Input: dimensioned drawing with shaded views. Units: mm. Origin: part minimum x, y, z. A direction names the side the tool comes from. Coordinates: 2 decimals unless noted, no trailing zeros. Write each loop counter-clockwise with the first axis right and the second up, starting at its lowest first coordinate (ties: lowest second). Pieces come first, ordered by that corner, then holes. Notation, with made-up numbers: M 15,84.5 L 38,84.5 A16 ccw 38,101.5 Z; hole C -16,75 d11. An arc over 180 degrees is marked long. Use one line per item in the form item = value.
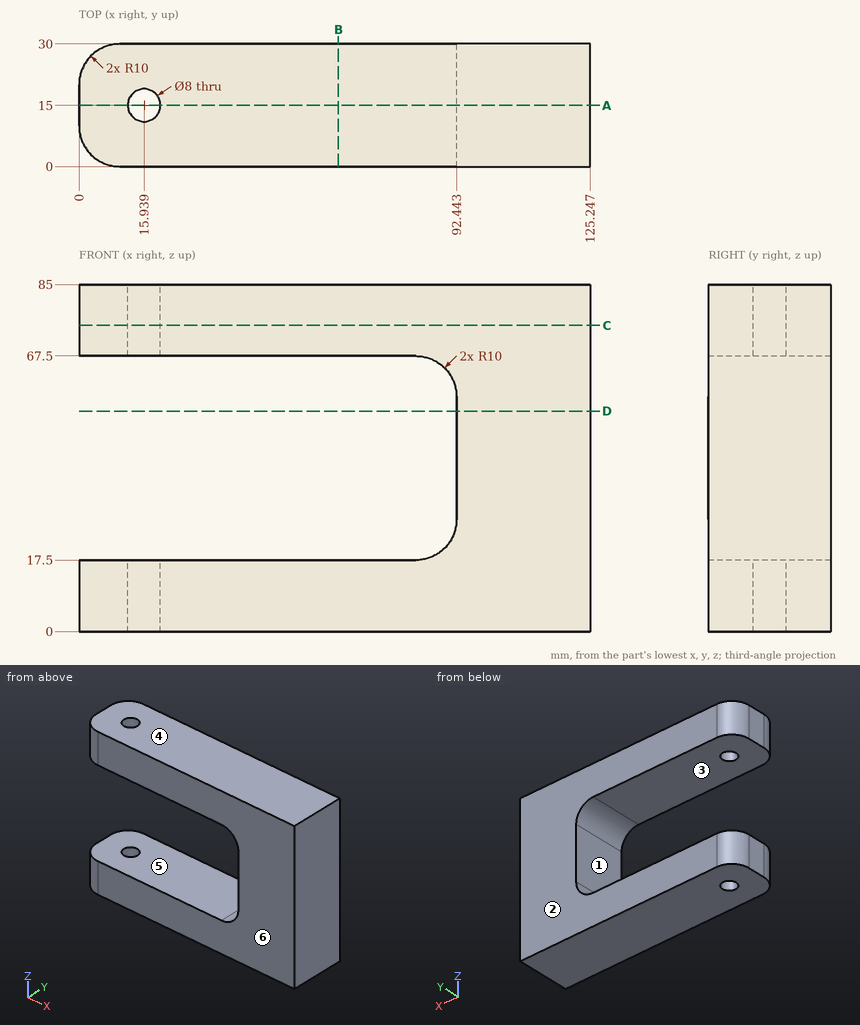
(1) Section query B-B on x = 63.5. Return the cut outline in (y, z).
Computed:
outline = M 0,0 L 30,0 L 30,17.5 L 0,17.5 Z; M 0,67.5 L 30,67.5 L 30,85 L 0,85 Z
(2) Pull-direction query (Z, two-part tool) for the marked faces 1, 2, 3 and 4; classes: pulls with the +Z half, pulls with the -Z half, needs draft (parallel to the pull), parting line crosses it, or undercut.
Computed:
face_1 = undercut
face_2 = needs draft
face_3 = undercut
face_4 = pulls with the +Z half
(3) Set-up query: the marked faces 5 and 6. Return all of +Z, -Z, +X, -X, +Y, -Y with unobstructed straight access to the full face (end or side cutting, diameter ignored); none if empty.
Computed:
face_5 = -X, +Y, -Y
face_6 = +Z, -Z, +X, -X, -Y
(4) Section query C-C on z = 75. Return the cut outline in (x, y).
Computed:
outline = M 0,10 A10 ccw 10,0 L 125.25,0 L 125.25,30 L 10,30 A10 ccw 0,20 Z; hole C 15.94,15 d8
(5) First-contact query: pin 1 Ø9 at (y, z) = (16.5, 37.5) entering from -X. Flat tip, straight axial feed; report the tip coordinate or a pass-through.
Computed:
pin_1 = 92.44
(6) Line query: probe 1 along Z at (x, y) = (63.5, 14.5); probe 2 along X at (y, z) = (17.25, 43.5); probe 3 along Y at (x, z) = (17, 4.5). Output: solid intervals per line, ascending.
Computed:
probe_1 = 0 to 17.5, 67.5 to 85
probe_2 = 92.44 to 125.25
probe_3 = 0 to 11.14, 18.86 to 30
(7) Section query A-A on y = 15. Return the cut outline in (x, z).
Computed:
outline = M 0,0 L 11.94,0 L 11.94,17.5 L 0,17.5 Z; M 0,67.5 L 11.94,67.5 L 11.94,85 L 0,85 Z; M 19.94,0 L 125.25,0 L 125.25,85 L 19.94,85 L 19.94,67.5 L 82.44,67.5 A10 cw 92.44,57.5 L 92.44,27.5 A10 cw 82.44,17.5 L 19.94,17.5 Z
(8) Section query D-D on z = 54. Return the cut outline in (x, y).
Computed:
outline = M 92.44,0 L 125.25,0 L 125.25,30 L 92.44,30 Z
